Autodesk Inventor part; units mm, degrees
ref_plane "YZ Plane" through (0, 0, 0) normal (1, 0, 0) x (0, 1, 0)
ref_plane "XZ Plane" through (0, 0, 0) normal (0, 1, 0) x (-1, 0, 0)
ref_plane "XY Plane" through (0, 0, 0) normal (0, 0, 1) x (1, 0, 0)
sketch "スケッチ1" plane through (0, 0, 0) normal (0, 0, 1) x (1, 0, 0)
  circle A0 centre (0, 0) radius 2
  dimension "d0" = 4
extrude "押し出し1" add sketch "スケッチ1" along normal blind 6
sketch "スケッチ2" plane through (0, 0, 6) normal (0, 0, 1) x (1, 0, 0)
  circle A0 centre (0, 0) radius 2
  circle A1 centre (0, 0) radius 4
  dimension "d3" = 8
extrude "押し出し2" add sketch "スケッチ2" along normal blind 2.3 contours A0 | A1
thread "ねじ1"
sketch "スケッチ3" plane through (0, 0, 0) normal (0, 0, -1) x (-1, 0, 0)
  circle A0 centre (0, 0) radius 2
extrude "押し出し3" cut sketch "スケッチ3" against normal blind 2.3
chamfer "面取り1" distance 2 angle 45 1 edges at (-4, 0, 6)
properties part number "SB　M4 6mm 皿ネジ" material "Stainless Steel, 440C"
Model file for the job. Use its own axes, mm. Round coordinates to 2 decimals unless told otherwise and drop trailing zeros. Write each loop counter-clockwise with the first axis right and the second up, starting at its lowest first coordinate (ties: lowest second). Pieces come first, ordered by that corner, then holes. Notation, with made-up numbers: (-33.75, -17) - (24.25, -17) arc R19 cw to (24.25, 15) - close; hole circle Ø9 at (-13, 40). An arc over 180 degrees is marked (long way). Use CSV: the item, a comma, the result in double quotes. Start each with the question number.
Item 1: Band-saw the part on C-C (z = 5.25). Write the cut outline in (x, y), and give its area (3 significant figures).
Item 2: Two-plate mould, pull along Y, no slides. Class faces 1 (the face through (0, 2, 4)), 2 (the face through (0, 0, 8.3)): released by +Y, released by -Y, zero draft, split by the parting line, or undercut.
Item 3: Pin check, flat tips, straight feed: P1, Ø1.5, axis at y = 0, z = 4, coming from the +X side; P2, Ø4, axis at x = 1, y = -2, coming from the -Z side; P3, Ø1.5, axis at x = 1, z = 7.5, coming from the +Y side; P4, Ø1.5, axis at y = 1.5, z = 3.5, coming from the +X side. Stop position of each tip, or through.
Item 4: Drill centre lines: L1, parallel to Z at x = -3, y = 2.5; L2, parallel to Z at x = 3.25, y = -2; L3, parallel to X at y = -1, z = 4.5. Where is each one in solid material? Low to high. Write a range as [from, to].
Checked values:
1,outline,"circle Ø4 at (0, 0)"
1,area,"12.6 mm²"
2,face 1,"split by the parting line"
2,face 2,"zero draft"
3,P1,"stops at x = 2"
3,P2,"stops at z = 2.3"
3,P3,"stops at y = 3.98"
3,P4,"stops at x = 1.85"
4,L1,"z = [7.9, 8.3]"
4,L2,"z = [7.82, 8.3]"
4,L3,"x = [-1.73, 1.73]"
